The model under review builds one solid part; all positions refer to its coordinate system, in mm. A direction names the side the tool comes from. Give positions to 0.01 mm unless a question says otherwise; leave off trailing zeros. Order: outer loops, then holes, each group sorted by start corner. A loop starts at its lowest first (then second) coordinate and runs counter-clockwise, first axis right, second up. Notation, with made-up numbers: (89.5, 87.5) -> (105.5, 87.5) arc R36 cw to (105.5, 122.5) -> close; hole circle Ø3 at (6.5, 82). An arc over 180 degrees is marked (long way). Use one line per item in the form item = value.
Autodesk Inventor part; units mm, degrees
ref_plane "YZ Plane" through (0, 0, 0) normal (1, 0, 0) x (0, 1, 0)
ref_plane "XZ Plane" through (0, 0, 0) normal (0, 1, 0) x (-1, 0, 0)
ref_plane "XY Plane" through (0, 0, 0) normal (0, 0, 1) x (1, 0, 0)
sketch "Sketch1" plane through (0, 0, 0) normal (0, 1, 0) x (-1, 0, 0)
  circle A0 centre (0, 0) radius 5
  circle A1 centre (0, 0) radius 10
  dimension "d0" = 10
  dimension "d1" = 20
extrude "Extrusion1" add sketch "Sketch1" along normal blind 16.5
sketch "Sketch2" plane through (0, 0, 0) normal (0, -1, 0) x (1, 0, 0)
  circle A0 centre (0, 0) radius 12.5
  circle A1 centre (0, 0) radius 10
  dimension "d4" = 25
extrude "Extrusion2" add sketch "Sketch2" against normal blind 5
fillet "Fillet1" radius 2 1 edges at (10, 16.5, 0)
properties part number "Bushing_beam" material "Brass, Soft Yellow"
1. Add section D-D on z = -11. Give the boundary of the cut face in (x, y).
Values:
outline = (-5.94, 0) -> (5.94, 0) -> (5.94, 5) -> (-5.94, 5) -> close
2. Tool access review of faces 4 (the face through (-0.2, 0, -5.4)), 5 (the face through (2.17, 9.68, 9.76)): name each direction out of +Z, -Z, +X, -X, +Y, -Y from which nothing blocks a thin tool from reaching the whole face with its end or side.
Values:
face_4 = +Z, -Z, +X, -X, -Y
face_5 = +Y
3. The part is to be moulded in two halves that separate along Z. For faces 1 (the face through (1.08, 8.13, 4.88)), 2 (the face through (0.1, 16.5, -5.2)), 3 (the face through (11.923, 2.465, 3.755)), say which applies: +Z half, -Z half, draft (parallel to the pull), parting line (faces both ways), or undercut.
Values:
face_1 = undercut
face_2 = draft
face_3 = parting line
4. Add section A-A on x = 0. Give the boundary of the cut face in (y, z), then the cut area to 3 significant figures.
Values:
outline = (0, -12.5) -> (5, -12.5) -> (5, -10) -> (14.5, -10) arc R2 ccw to (16.5, -8) -> (16.5, -5) -> (0, -5) -> close; (0, 5) -> (16.5, 5) -> (16.5, 8) arc R2 ccw to (14.5, 10) -> (5, 10) -> (5, 12.5) -> (0, 12.5) -> close
area = 188 mm^2
5. Add section C-C on y = 3.25. Give the boundary of the cut face in (x, z), then the cut area to 3 significant figures.
Values:
outline = circle Ø25 at (0, 0); hole circle Ø10 at (0, 0)
area = 412 mm^2
6. For L1, parallel to Z at x = 0, y = 9.5; L2, parallel to Z at x = 0, y = 4.25; L3, parallel to Y at x = -4.75, z = 9.5, list the stretches that pass through material, from the lowest coordinate up.
Values:
L1 = -10 to -5, 5 to 10
L2 = -12.5 to -5, 5 to 12.5
L3 = 0 to 5
7. Add section B-B on z = 0. Give the boundary of the cut face in (x, y), then the cut area to 3 significant figures.
Values:
outline = (-12.5, 0) -> (-5, 0) -> (-5, 16.5) -> (-8, 16.5) arc R2 ccw to (-10, 14.5) -> (-10, 5) -> (-12.5, 5) -> close; (5, 0) -> (12.5, 0) -> (12.5, 5) -> (10, 5) -> (10, 14.5) arc R2 ccw to (8, 16.5) -> (5, 16.5) -> close
area = 188 mm^2
8. For pin 1 Ø9 at (x, z) = (0, 0) entering from +Y; pin 2 Ø3 at (y, z) = (8.5, -5.5) entering from +X; pin 3 Ø1 at (y, z) = (6.5, -2) entering from -X; pin 4 Ø3 at (x, y) = (6, 14.5) entering from -Z, all flat-tipped, find the tip position at first contact; note any pin that passes through.
Values:
pin_1 = through
pin_2 = 9.17
pin_3 = -9.89
pin_4 = -8.93
